Autodesk Inventor part; units mm, degrees
ref_plane "Work Plane2" through (0, 0, 3) normal (0, 0, 1) x (1, 0, 0)
ref_plane "Work Plane3" through (3, 0, 0) normal (1, 0, 0) x (0, 1, 0)
ref_plane "XZ Plane" through (0, 0, 0) normal (0, 1, 0) x (-1, 0, 0)
sketch "Sketch1" plane through (0, 0, 0) normal (0, 1, 0) x (-1, 0, 0)
  circle A0 centre (0, 0) radius 3
  dimension "d0" = 6
extrude "Extrusion1" add sketch "Sketch1" along normal blind 10
fillet "Fillet1" radius 3 1 edges at (3, 10, 0)
ref_plane "Work Plane2" through (0, 0, 3) normal (0, 0, 1) x (1, 0, 0)
ref_plane "Work Plane3" through (3, 0, 0) normal (1, 0, 0) x (0, 1, 0)
sketch "Sketch6" plane through (3, 0, 0) normal (1, 0, 0) x (0, 1, 0)
  circle A0 centre (7, 0) radius 1.5
  arc A1 (7, -3) -> (7, 3) centre (7, 0) ccw
  point P0 (0, 0)
  dimension "d21" = 3
extrude "Extrusion4" cut sketch "Sketch6" against normal blind 6
sketch "Sketch5" plane through (0, 0, 3) normal (0, 0, 1) x (1, 0, 0)
  line L0 (3, 0) -> (-3, 0)
  line L1 (-1.5, 9.5981) -> (-1.5, 3)
  line L2 (-1.5, 3) -> (1.5, 3)
  line L3 (1.5, 3) -> (1.5, 9.5981)
  arc A0 (2.5981, 8.5) -> (-2.5981, 8.5) centre (0, 7) ccw
  line L4 (0, 3) -> (0, 10) construction
  line L5 (2.5981, 7) -> (-2.5981, 7)
  arc A1 (1.4921, 9.6026) -> (-1.5, 9.5981) centre (0, 7) ccw
  point P0 (0, 0)
  point P1 (3, 10)
  point P2 (-3, 10)
  point P3 (0, 9.7895)
  point P4 (0, 10)
  point P5 (0, 0)
  dimension "d16" = 3
  dimension "d25" = 7
  dimension "d26" = 1.5
extrude "Extrusion3" cut sketch "Sketch5" against normal blind 6
sketch "Sketch7" plane through (0, 0, 0) normal (0, -1, 0) x (1, 0, 0)
  circle A0 centre (0, 0) radius 3
hole "Hole2" at (0, 0, 0) direction (0, 1, 0) diameter 2.459 depth 3
properties part number "19.1"
Can you work these out from the model? Positions are in its coordinate system, mm. A direction names the side the tool comes from. Give positions to 0.01 mm unless a question says otherwise; leave off trailing zeros. Order: outer loops, then holes, each group sorted by start corner. A loop starts at its lowest first (then second) coordinate and runs counter-clockwise, first axis right, second up. Notation, with made-up numbers: M 58,45 L 76,45 A32 ccw 76,73 Z; hole C 66.25,77 d3. An arc over 180 degrees is marked long. Use a Markdown table: item, result. Add a question column.
Item 1: Suppose I cut it at C-C (y = 6.25). List the corners of the cut face in (x, z) for me.
Item 2: Suppose I cut it at B-B (x = 0). List the corners of the cut face in (y, z) for me, then the cut area to 3 significant figures.
Item 3: We'd pull the mould along X, two halves only. Please class faces 3 (the flat face through (-1, 0, -1)), 4 (the cylindrical face through (0.748, 1.521, 0.976)), 5 (the cylindrical face through (0.391, 2.673, -2.974)): +X half, -X half, draft (parallel to the pull), parting line (faces both ways), or undercut.
Item 4: For faces 1 (the cylindrical face through (2.09, 5.5, 0.07)), 2 (the flat face through (-1.5, 5, 0)), which set-ups out of +Z, -Z, +X, -X, +Y, -Y let a thin tool reach every point of the face, with its end or its side?
Item 5: If I drill on L1, parallel to X at y = 3.25, z = 0; L2, parallel to X at y = 2.25, z = 0, over which ranges is the centre line in solid material (lowest first)? Write a range as [from, to].
Item 6: Will these pins go through, and if not, where does the flat tip stop? pin 1 (3.5 mm diameter, centred on x = 0, z = 0.5, fed in from +Y); pin 2 (1.5 mm diameter, centred on y = 2.5, z = -2, fed in from -X); pin 3 (1.5 mm diameter, centred on x = -1.5, z = -2, fed in from +Y); pin 4 (3 mm diameter, centred on x = -2, y = 8, fed in from +Z).
Item 7: Suppose I cut it at A-A (z = 0). List the corners of the cut face in (x, y) for me, then the cut area to 3 significant figures.
Item 8: Suppose I cut it at D-D (y = 4.75). List the corners of the cut face in (x, z) for me, then the cut area to 3 significant figures.
Answer sheet:
| question | item | result |
|---|---|---|
| 1 | outline | M -2.7,-1.3 A3 ccw -1.5,-2.6 L -1.5,-1.3 Z; M -2.7,1.3 L -1.5,1.3 L -1.5,2.6 A3 ccw Z; M 1.5,-2.6 A3 ccw 2.7,-1.3 L 1.5,-1.3 Z; M 1.5,1.3 L 2.7,1.3 A3 ccw 1.5,2.6 Z |
| 2 | outline | M 0,-3 L 3,-3 L 3,-1.23 L 0,-1.23 Z; M 0,1.23 L 3,1.23 L 3,3 L 0,3 Z |
| 2 | area | 10.6 mm² |
| 3 | face 3 | draft |
| 3 | face 4 | undercut |
| 3 | face 5 | parting line |
| 4 | face 1 | +X, -X |
| 4 | face 2 | +Z, -Z, +Y |
| 5 | L1 | x = [-3, -1.5], [1.5, 3] |
| 5 | L2 | x = [-3, -1.23], [1.23, 3] |
| 6 | pin 1 | stops at y = 9.6 |
| 6 | pin 2 | stops at x = -2.73 |
| 6 | pin 3 | stops at y = 9.28 |
| 6 | pin 4 | stops at z = 2.6 |
| 7 | outline | M -3,0 L -1.23,0 L -1.23,3 L -1.5,3 L -1.5,5.5 L -3,5.5 Z; M -2.6,8.5 L -1.5,8.5 L -1.5,9.6 A3 ccw Z; M 1.23,0 L 3,0 L 3,5.5 L 1.5,5.5 L 1.5,3 L 1.23,3 Z; M 1.5,8.5 L 2.6,8.5 A3 ccw 1.5,9.6 Z |
| 7 | area | 19.5 mm² |
| 8 | outline | M -1.5,-2.6 L -1.5,2.6 A3 ccw Z; M 1.5,-2.6 A3 ccw 1.5,2.6 Z |
| 8 | area | 11.1 mm² |
